For this review, take the finished solid that the model builds, in its own axes (mm). A direction names the side the tool comes from. Give positions to 0.01 mm unless a question says otherwise; leave off trailing zeros. Order: outer loops, then holes, each group sorted by start corner. A loop starts at its lowest first (then second) coordinate and runs counter-clockwise, first axis right, second up. Notation, with made-up numbers: (-3.75, 64) - (48.25, 64) arc R17 cw to (48.25, 74) - close; hole circle Ø2 at (14.25, 9). An arc over 180 degrees is marked (long way). One line per item, written item: value.
```python
from build123d import *

# Parameters (mm, degrees)
SKETCH12_R          = 2.75
BOSS_EXTRUDE5_DEPTH = 2
BOSS_EXTRUDE6_START = -1
SKETCH20_R          = 3.25
BOSS_EXTRUDE6_DEPTH = 2
SKETCH21_W          = 6.2
SKETCH21_H          = 2
BOSS_EXTRUDE7_DEPTH = 2
BOSS_EXTRUDE8_DEPTH = 2
FILLET1_R           = 1


with BuildPart() as part:
    # Sketch12 → Boss-Extrude5 (new body)
    with BuildSketch(Plane(origin=(0, 0, 0), x_dir=(1, 0, 0), z_dir=(0, 1, 0))):
        with BuildLine():
            Line((0, 5), (-5, 5))
            Line((-5, 5), (-5, -5))
            Line((-5, -5), (0, -5))
            ThreePointArc((0, -5), (5, 0), (0, 5))
        make_face()
        with Locations(Location((0, 0, 0), (0, 0, 270))):
            Circle(SKETCH12_R, mode=Mode.SUBTRACT)
    extrude(amount=BOSS_EXTRUDE5_DEPTH)

    # Sketch21 → Boss-Extrude7 (add)
    with BuildSketch(Plane.XZ):
        with BuildLine():
            Line((-5, -5), (-6, -5))
            Line((-6, -5), (-12.2, -5))
            ThreePointArc((-12.2, -5), (-13.614213562, -4.414213562), (-14.2, -3))
            Line((-14.2, -3), (-14.2, -1))
            ThreePointArc((-14.2, -1), (-13.956204356, -0.043053679), (-13.28425374, 0.680593296))
            Line((-13.28425374, 0.680593296), (-7.08425374, 4.680593296))
            ThreePointArc((-7.08425374, 4.680593296), (-6.565160777, 4.918487242), (-6, 5))
            Line((-6, 5), (-5, 5))
            Line((-5, 5), (-5, -5))
        make_face()
        with Locations((-9.1, -2)):
            Rectangle(SKETCH21_W, SKETCH21_H, mode=Mode.SUBTRACT)
    extrude(amount=-BOSS_EXTRUDE7_DEPTH)



with BuildPart() as body_2:
    # Sketch20 → Boss-Extrude6 (new body)
    with BuildSketch(Plane.XY.offset(BOSS_EXTRUDE6_START)):
        with BuildLine():
            Line((-15.2, -8.4), (-15.2, 1.6))
            Line((-15.2, 1.6), (-30.2, 1.6))
            ThreePointArc((-30.2, 1.6), (-35.2, -3.4), (-30.2, -8.4))
            Line((-30.2, -8.4), (-15.2, -8.4))
        make_face()
        with Locations((-30.2, -3.4)):
            Circle(SKETCH20_R, mode=Mode.SUBTRACT)
    extrude(amount=-BOSS_EXTRUDE6_DEPTH)


with BuildPart() as part_1:
    add(part.part)

    add(body_2.part)  # Boss-Extrude8 merges body 2
    # Sketch22 → Boss-Extrude8 (add)
    with BuildSketch(Plane.XY.offset(-1)):
        with BuildLine():
            Line((-6.648176396, -1.473965041), (-13.626436158, -7.873965041))
            ThreePointArc((-13.626436158, -7.873965041), (-14.252977088, -8.26385757), (-14.978259763, -8.4))
            Line((-14.978259763, -8.4), (-15.2, -8.4))
            Line((-15.2, -8.4), (-15.2, 1.6))
            Line((-15.2, 1.6), (-6, 1.6))
            Line((-6, 1.6), (-6, 0))
            ThreePointArc((-6, 0), (-6.169201375, -0.805094029), (-6.648176396, -1.473965041))
        make_face()
    extrude(amount=-BOSS_EXTRUDE8_DEPTH)

    # Fillet1
    fillet1_edges = [part_1.edges().sort_by_distance(p)[0] for p in [
        (-6, 0, -2),
        (-14.2, 0.8, -1),
        (-14.2, 0.8, -3),
        (-10.1, 0, -3),
        (-10.1, 0, -1),
    ]]
    fillet(fillet1_edges, radius=FILLET1_R)


solid = part_1.part
```
(1) Take a section at C-C (x = -20). Write out the cut boundary in (y, z), then the cut area to 3 significant figures.
Answers below:
outline: (-8.4, -3) - (1.6, -3) - (1.6, -1) - (-8.4, -1) - close
area: 20.0 mm^2
(2) Draft analysis for pull direction X (two halves, no side actions). For faces 1 (the face through (-22, 1.6, -2)), 2 (the face through (-2.685, 0.986, -0.596)), 3 (the face through (5, 1, 0)), state which applies: pulls with the +X half, pulls with the -X half, needs draft (parallel to the pull), parting line crosses it, or undercut.
Answers below:
face 1: needs draft
face 2: undercut
face 3: pulls with the +X half
(3) Take a section at D-D (y = -7.25). Write out the cut boundary in (x, z), then the cut area to 3 significant figures.
Answers below:
outline: (-33.39, -3) - (-12.95, -3) - (-12.95, -1) - (-33.39, -1) - close
area: 40.9 mm^2
(4) Machinability: for faces 4 (the face through (-3, 1, 5)), 5 (the face through (-21, -3, -1)), 6 (the face through (-14.44, 0.61, -0.81)), 7 (the face through (-21, -3, -3)), 8 (the face through (-9, 1.6, -2)), which of the approach directions +Z, -Z, +X, -X, +Y, -Y give a long, thin tool a straight path to every point of the face, cutting with its end or side? Answer none if there is none.
Answers below:
face 4: +Z, +X, -X, +Y, -Y
face 5: +Z, -X, -Y
face 6: +Z, -X, +Y, -Y
face 7: -Z, -X, -Y
face 8: +Y
(5) Take a section at B-B (y = -3.4). Write out the cut boundary in (x, z).
Answers below:
outline: (-35.2, -3) - (-33.45, -3) - (-33.45, -1) - (-35.2, -1) - close; (-26.95, -3) - (-8.75, -3) - (-8.75, -1) - (-26.95, -1) - close
(6) Wall thickness on line 1 (X direction, y = 0.9, z = 0); line 2 (Z direction, x = -32, y = -6.75); line 3 (X direction, y = 0.5, z = -0.25): over which ranges is each line inside the solid? List them lowest first. Write a range as from..to.
Answers below:
line 1: x = -13.93..-2.75, 2.75..5
line 2: z = -3..-1
line 3: x = -14.05..-2.74, 2.74..4.99
(7) For P1, Ø2, axis at y = -2, z = 1.5, coming from the +X side; P2, Ø2.5, axis at x = -24, z = -2, coming from the +Y side; P3, Ø5, axis at x = -14.5, y = -4, coming from the +Z side; P4, Ø5, axis at x = -5, z = 2.5, coming from the -Y side, all flat-tipped, find the tip position at first contact; note any pin that passes through.
Answers below:
P1: passes through
P2: stops at y = 1.6
P3: stops at z = -1
P4: stops at y = 0
(8) Take a section at A-A (x = 0.5). Write out the cut boundary in (y, z), then the cut area to 3 significant figures.
Answers below:
outline: (0, -4.97) - (2, -4.97) - (2, -2.7) - (0, -2.7) - close; (0, 2.7) - (2, 2.7) - (2, 4.97) - (0, 4.97) - close
area: 9.08 mm^2
